Design review of the part built by this model. Coordinates are the model's own, in mm. A direction names the side the tool comes from. Coordinates: 2 decimals unless noted, no trailing zeros. Loops run counter-clockwise (first coordinate to the right, second up) from the corner with the lowest first, then second, coordinate; pieces in that order, holes last. Notation, with made-up numbers: M -33,-8 L -27,-8 A12 ccw -27,13 Z; hole C -35,-18.5 d5. An arc over 180 degrees is marked long. Answer as a JSON object with one key per item and string values. Group by question number.
1. Consider section B-B (y = 4.5). State the section outline as (x, z) points.
2. Insertion check: pin 1 (3 mm diameter, centred on x = 2.5, y = 0.5, fed in from -Z); pin 2 (1.5 mm diameter, centred on x = 18, y = -2, fed in from +Z). Each pin has a flat end and moves straight along its axis. Give the tip position at first contact, or say it passes through.
3. To check wall thickness, follow probe 1 along Y at (x, z) = (12.5, 2); probe 2 along X at (y, z) = (4, 3); probe 3 along Y at (x, z) = (14.5, 6). State the ranges of each line that lie inside material, in increasing order.
4. Consider section D-D (x = 12). State the section outline as (y, z) points.
5. Draft analysis for pull direction X (two halves, no side actions). For faces 1 (the flat face through (48, 0, 3)), 2 (the flat face through (-1, 10, 4)), 3 (the flat face through (-48, 0, 3)), 4 (the flat face through (1, 11, 3)), state which applies: +X half, -X half, draft (parallel to the pull), parting line (faces both ways), or undercut.
6. Machinability: for faces 5 (the flat face through (-1, -11, 3)), 6 (the flat face through (-0.2, 8.2, 1)), which of the approach directions +Z, -Z, +X, -X, +Y, -Y give a long, thin tool a straight path to every point of the face, cutting with its end or side? Answer none if there is none.
7. Consider section A-A (z = 2). Count the separate pieces of the cut face and the enclosed holes in it, then the cut area to 3 significant figures.
Autodesk Inventor part; units mm, degrees
ref_plane "YZ Plane" through (0, 0, 0) normal (1, 0, 0) x (0, 1, 0)
ref_plane "XZ Plane" through (0, 0, 0) normal (0, 1, 0) x (-1, 0, 0)
ref_plane "XY Plane" through (0, 0, 0) normal (0, 0, 1) x (1, 0, 0)
sketch "Sketch2" plane through (0, 0, 0) normal (0, 0, 1) x (1, 0, 0)
  line L0 (-46, 10) -> (46, 10)
  line L1 (47, 9) -> (47, -9)
  line L2 (46, -10) -> (-46, -10)
  line L3 (-47, -9) -> (-47, 9)
  line L4 (-47, 10) -> (47, -10) construction
  line L5 (47, 10) -> (-47, -10) construction
  line L6 (45, 8) -> (-45, 8)
  line L7 (-45, 8) -> (-45, -8)
  line L8 (-45, -8) -> (45, -8)
  line L9 (45, -8) -> (45, 8)
  line L10 (48, 11) -> (-48, 11)
  line L11 (-48, 11) -> (-48, -11)
  line L12 (-48, -11) -> (48, -11)
  line L13 (48, -11) -> (48, 11)
  arc A0 (47, 9) -> (46, 10) centre (46, 9) ccw
  arc A1 (46, -10) -> (47, -9) centre (46, -9) ccw
  arc A2 (-47, -9) -> (-46, -10) centre (-46, -9) ccw
  arc A3 (-46, 10) -> (-47, 9) centre (-46, 9) ccw
  point P0 (0, 0)
  dimension "d0" = 94
  dimension "d1" = 20
  dimension "d2" = 2
  dimension "d3" = 1
  dimension "d10" = 1
  dimension "d40" = 90
extrude "Extrusion1" add sketch "Sketch2" along normal blind 1 contours L0 A0 L1 A1 L2 A2 L3 A3 | L9 L8 L7 L6 | L13 L12 L11 L10
extrude "Extrusion2" add sketch "Sketch2" along normal blind 7 contours L13 L12 L11 L10
extrude "Extrusion3" add sketch "Sketch2" along normal blind 4 contours L9 L8 L7 L6
sketch "Sketch4" plane through (-48, -11, 0) normal (0, -1, 0) x (1, 0, 0)
  circle A0 centre (22.1132, 6) radius 0.5
  circle A1 centre (29.8868, 6) radius 0.5
  circle A2 centre (44.1132, 6) radius 0.5
  circle A3 centre (51.8842, 6) radius 0.5
  circle A4 centre (66.1132, 6) radius 0.5
  circle A5 centre (73.8868, 6) radius 0.5
  line L0 (0, 6) -> (96, 6)
  line L1 (96, 7) -> (0, 7)
  line L2 (22.1132, 4) -> (22.1132, 4)
  line L3 (22.6132, 4.5) -> (22.6132, 8)
  line L4 (22.6132, 8) -> (21.6132, 8)
  line L5 (21.6132, 8) -> (21.6132, 4.5)
  line L6 (21.6132, 4) -> (22.6132, 8) construction
  line L7 (22.6132, 4) -> (21.6132, 8) construction
  line L8 (29.8868, 4) -> (29.8868, 4)
  line L9 (30.3868, 4.5) -> (30.3868, 8)
  line L10 (30.3868, 8) -> (29.3868, 8)
  line L11 (29.3868, 8) -> (29.3868, 4.5)
  line L12 (29.3868, 4) -> (30.3868, 8) construction
  line L13 (30.3868, 4) -> (29.3868, 8) construction
  line L14 (44.1132, 4) -> (44.1132, 4)
  line L15 (44.6132, 4.5) -> (44.6132, 8)
  line L16 (44.6132, 8) -> (43.6132, 8)
  line L17 (43.6132, 8) -> (43.6132, 4.5)
  line L18 (43.6132, 4) -> (44.6132, 8) construction
  line L19 (44.6132, 4) -> (43.6132, 8) construction
  line L20 (51.8842, 4) -> (51.8842, 4)
  line L21 (52.3842, 4.5) -> (52.3842, 8)
  line L22 (52.3842, 8) -> (51.3842, 8)
  line L23 (51.3842, 8) -> (51.3842, 4.5)
  line L24 (51.3842, 4) -> (52.3842, 8) construction
  line L25 (52.3842, 4) -> (51.3842, 8) construction
  line L26 (66.1132, 4) -> (66.1132, 4)
  line L27 (65.6132, 4.5) -> (65.6132, 8)
  line L28 (65.6132, 8) -> (66.6132, 8)
  line L29 (66.6132, 8) -> (66.6132, 4.5)
  line L30 (66.6132, 4) -> (65.6132, 8) construction
  line L31 (65.6132, 4) -> (66.6132, 8) construction
  line L32 (73.8868, 4) -> (73.8868, 4)
  line L33 (73.3868, 4.5) -> (73.3868, 8)
  line L34 (73.3868, 8) -> (74.3868, 8)
  line L35 (74.3868, 8) -> (74.3868, 4.5)
  line L36 (74.3868, 4) -> (73.3868, 8) construction
  line L37 (73.3868, 4) -> (74.3868, 8) construction
  arc A6 (21.6132, 4.5) -> (22.1132, 4) centre (22.1132, 4.5) ccw
  arc A7 (22.1132, 4) -> (22.6132, 4.5) centre (22.1132, 4.5) ccw
  arc A8 (29.3868, 4.5) -> (29.8868, 4) centre (29.8868, 4.5) ccw
  arc A9 (29.8868, 4) -> (30.3868, 4.5) centre (29.8868, 4.5) ccw
  arc A10 (43.6132, 4.5) -> (44.1132, 4) centre (44.1132, 4.5) ccw
  arc A11 (44.1132, 4) -> (44.6132, 4.5) centre (44.1132, 4.5) ccw
  arc A12 (51.3842, 4.5) -> (51.8842, 4) centre (51.8842, 4.5) ccw
  arc A13 (51.8842, 4) -> (52.3842, 4.5) centre (51.8842, 4.5) ccw
  arc A14 (65.6132, 4.5) -> (66.1132, 4) centre (66.1132, 4.5) ccw
  arc A15 (66.1132, 4) -> (66.6132, 4.5) centre (66.1132, 4.5) ccw
  arc A16 (73.3868, 4.5) -> (73.8868, 4) centre (73.8868, 4.5) ccw
  arc A17 (73.8868, 4) -> (74.3868, 4.5) centre (73.8868, 4.5) ccw
  point P0 (96, 0)
  point P1 (69, 6)
  point P2 (71, 6)
  point P3 (49, 6)
  point P4 (47, 6)
  point P5 (27, 6)
  point P6 (25, 6)
  point P7 (22.1132, 4)
  dimension "d59" = 1
  dimension "d60" = 1
  dimension "d61" = 1
  dimension "d62" = 1
  dimension "d63" = 1
  dimension "d64" = 1
  dimension "d65" = 1
  dimension "d66" = 4
  dimension "d67" = 1
  dimension "d68" = 4
  dimension "d69" = 1
  dimension "d70" = 4
  dimension "d71" = 1
  dimension "d72" = 4
  dimension "d73" = 1
  dimension "d74" = 4
  dimension "d75" = 1
  dimension "d76" = 4
  dimension "d81" = 0.5
sketch "Sketch3" plane through (0, 0, 4) normal (0, 0, 1) x (1, 0, 0)
  line L0 (-53.1158, -1) -> (46.8842, -1) construction
  line L1 (43, 0) -> (23, 0) construction
  line L2 (23, 0) -> (23, 5) construction
  line L3 (23, 5) -> (43, 5) construction
  line L4 (43, 5) -> (43, 0) construction
  line L5 (23, 0) -> (23, 5.2137) construction
  line L6 (43, 0) -> (40.1132, 5) construction
  line L7 (46.8842, -1) -> (46.8842, 4.7735) construction
  line L8 (23, 0) -> (25.8868, 5) construction
  line L9 (23, 0) -> (23, 4.6279) construction
  line L10 (21, 0) -> (18.1132, 5) construction
  line L11 (1, 5) -> (21, 5) construction
  line L12 (1, 0) -> (3.8868, 5) construction
  line L13 (-1, 0) -> (-3.8868, 5) construction
  line L14 (-21, 5) -> (-1, 5) construction
  line L15 (-21, 0) -> (-18.1132, 5) construction
  line L16 (-23, 0) -> (-25.8868, 5) construction
  line L17 (-43, 5) -> (-23, 5) construction
  line L18 (-43, 0) -> (-40.1132, 5) construction
  line L19 (43, 5) -> (-43, 5) construction
  line L20 (0, 5) -> (0, 5) construction
  circle A0 centre (-25.8868, 0) radius 0.5
  circle A1 centre (-18.1132, 0) radius 0.5
  circle A2 centre (-3.8868, 0) radius 0.5
  circle A3 centre (3.8842, 0) radius 0.5
  circle A4 centre (18.1132, 0) radius 0.5
  circle A5 centre (25.8868, 0) radius 0.5
  line L21 (-45, 8) -> (-45, -8)
  line L22 (45, -8) -> (45, 8)
  line L23 (-48, 11) -> (-48, -11)
  line L24 (-48, 0) -> (48, 0)
  line L25 (48, -11) -> (48, 11)
  point P0 (3.8842, 4)
  dimension "d45" = 20
  dimension "d46" = 5
  dimension "d47" = 30
  dimension "d48" = 30
  dimension "d49" = 22
  dimension "d52" = 0
  dimension "d53" = 1
  dimension "d54" = 1
  dimension "d55" = 1
  dimension "d56" = 1
  dimension "d57" = 1
  dimension "d58" = 1
extrude "Extrusion4" cut sketch "Sketch4" against normal blind 10 contours L0 A0 | L3 A7 A6 L5 A0 | A0 L0 | A0 L5 L1 L3 | L11 L1 L9 A1 | L0 A1 | A1 L0 | A1 L9 A9 A8 L11 | L1 L5 L4 L3 | L11 L10 L9 L1 | L17 L1 L15 A2 | L0 A2 | A2 L0 | A2 L15 A11 A10 L17 | L17 L16 L15 L1 | L23 L1 L21 A3 | L0 A3 | A3 L0 | A3 L21 A13 A12 L23 | L23 L22 L21 L1 | L27 L1 L29 A4 | L0 A4 | A4 L0 | A4 L29 A15 A14 L27 | L27 L28 L29 L1 | L33 L1 L35 A5 | L0 A5 | A5 L0 | A5 L35 A17 A16 L33 | L33 L34 L35 L1
extrude "Extrusion5" cut sketch "Sketch3" against normal blind 10
properties part number "sdm_finger_eit_chamber_mould"
Findings below:
{
 "1": {"outline": "M -48,0 L 48,0 L 48,7 L 47,7 L 47,1 L 45,1 L 45,4 L -45,4 L -45,1 L -47,1 L -47,7 L -48,7 Z"},
 "2": {"pin 1": "stops at z = 0", "pin 2": "stops at z = 4"},
 "3": {"probe 1": "y = -11 to -10, -8 to 8, 10 to 11", "probe 2": "x = -48 to -47, -45 to 45, 47 to 48", "probe 3": "y = -11 to -10, 10 to 11"},
 "4": {"outline": "M -11,0 L 11,0 L 11,7 L 10,7 L 10,1 L 8,1 L 8,4 L -8,4 L -8,1 L -10,1 L -10,7 L -11,7 Z"},
 "5": {"face 1": "+X half", "face 2": "undercut", "face 3": "-X half", "face 4": "draft"},
 "6": {"face 5": "+Z, -Z, +X, -X, -Y", "face 6": "+Z"},
 "7": {"separate pieces": "2", "enclosed holes": "7", "area": "1,670 mm^2"}
}
